Input: dimensioned drawing with shaded views. Units: mm. Origin: part minimum x, y, z. A direction names the side the tool comes from. Round coordinates to 2 decimals unless told otherwise and drop trailing zeros. Write each loop counter-clockwise with the first axis right and the second up, starting at its lowest first coordinate (ties: lowest second). Pieces come first, ordered by that corner, then holes. Notation, with made-up numbers: (30, 84) - (70, 84) arc R18 ccw to (70, 107) - close; hole circle Ø10 at (-21, 53). An arc over 180 degrees is marked (long way). Use one line per item in the form item = value.
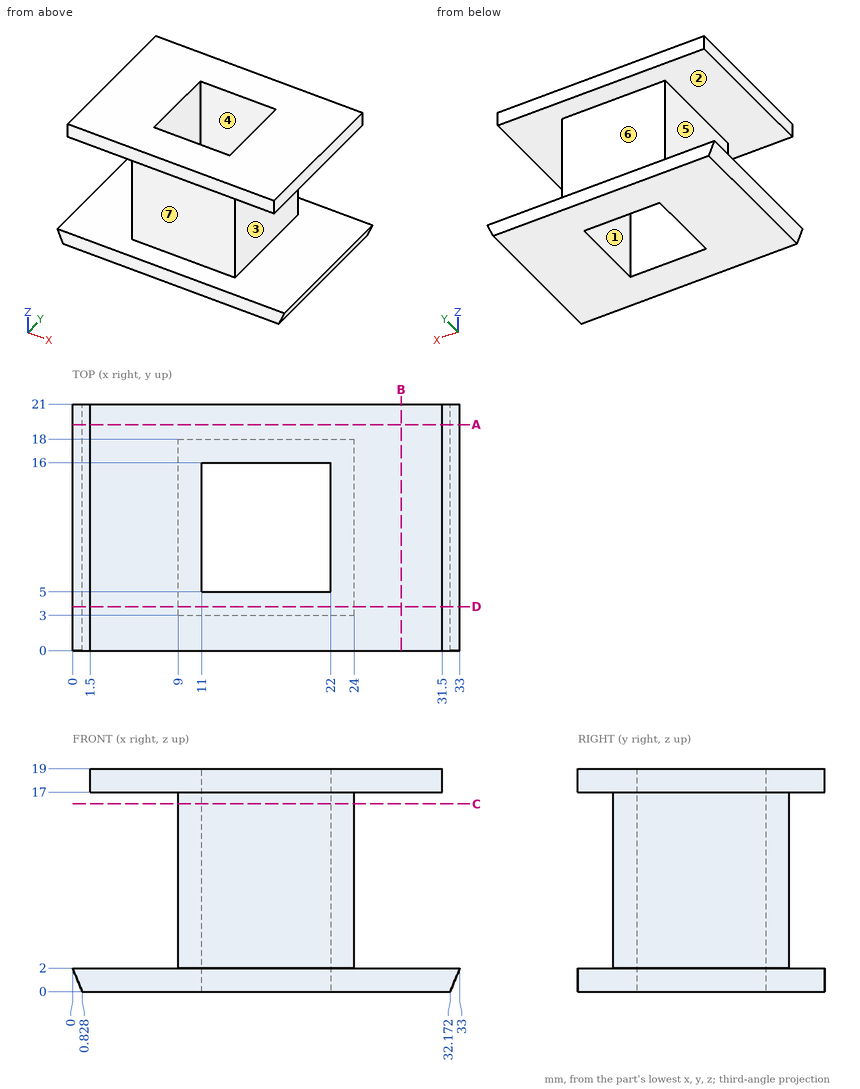
(1) Cut plane B-B on x = 28. Output: boundary loops of the cut face in (y, z).
Derived:
outline = (0, 0) - (21, 0) - (21, 2) - (0, 2) - close; (0, 17) - (21, 17) - (21, 19) - (0, 19) - close
(2) Access query for the marked faces 4, 5, 6 and 7. Directions: +Z, -Z, +X, -X, +Y, -Y. A direction counts if a zero-diameter tool reaches every point of the face in a straight line with its end or side. Return the directions, or none.
Derived:
face_4 = +Z, -Z
face_5 = -X, +Y, -Y
face_6 = +X, -X, +Y
face_7 = +X, -X, -Y
(3) Cut plane A-A on y = 19.25. Output: boundary loops of the cut face in (x, z).
Derived:
outline = (0, 2) - (0.83, 0) - (32.17, 0) - (33, 2) - close; (1.5, 17) - (31.5, 17) - (31.5, 19) - (1.5, 19) - close
(4) Draft query along X for the marked faces 1, 2 and 3. Return one class per face: released by +X, released by -X, zero draft, split by the parting line, or undercut.
Derived:
face_1 = undercut
face_2 = zero draft
face_3 = released by +X
(5) Cut plane C-C on z = 16. Output: boundary loops of the cut face in (x, y), then the cut area to 3 significant figures.
Derived:
outline = (9, 3) - (24, 3) - (24, 18) - (9, 18) - close; hole (11, 5) - (22, 5) - (22, 16) - (11, 16) - close
area = 104 mm^2
(6) First-contact query: pin 1 Ø0.6 at (y, z) = (14, 17.5) entering from -X; pin 2 Ø1.6 at (y, z) = (10.5, 18.5) entering from +X; pin 3 Ø3 at (x, z) = (13.5, 15) entering from -Y. Flat tips, straight axial feed; report the tip coordinate or a pass-through.
Derived:
pin_1 = 1.5
pin_2 = 31.5
pin_3 = 3
(7) Cut plane D-D on y = 3.75. Output: boundary loops of the cut face in (x, z), then the cut area to 3 significant figures.
Derived:
outline = (0, 2) - (0.83, 0) - (32.17, 0) - (33, 2) - (24, 2) - (24, 17) - (31.5, 17) - (31.5, 19) - (1.5, 19) - (1.5, 17) - (9, 17) - (9, 2) - close
area = 349 mm^2
(8) Material intervals for L1, parallel to Y at x = 13.5, z = 4; L2, parallel to Z at x = 5.5, y = 18.75; L3, parallel to X at y = 5.5, z = 5.75, sorted ascending.
Derived:
L1 = 3 to 5, 16 to 18
L2 = 0 to 2, 17 to 19
L3 = 9 to 11, 22 to 24
